Verification items for the finished model (mm, model axes). A direction names the side the tool comes from. Give positions to 0.01 mm unless a question says otherwise; leave off trailing zeros. Order: outer loops, then holes, each group sorted by start corner. A loop starts at its lowest first (then second) coordinate and runs counter-clockwise, first axis right, second up. Notation, with made-up numbers: M 43.5,79 L 72.5,79 A19 cw 72.5,108 Z; hole C 49,21.5 d9. An arc over 180 degrees is marked long. Answer as a JSON object with one key per item and string values.
```python
from build123d import *

# Parameters (mm, degrees)
BOSS_EXTRUDE1_DEPTH = 3


with BuildPart() as part:
    # Sketch1 → Boss-Extrude1 (new body)
    with BuildSketch(Plane(origin=(0, 0, 0), x_dir=(0, 0, -1), z_dir=(1, 0, 0))):
        Polygon((-23.405592815, -13.328738611), (32.192831055, -13.328738611), (32.192831055, -19.328738611), (34.462282484, -20.506092894), (31.699266712, -25.832042935), (36.137558413, -28.134556078), (38.900574185, -22.808606037), (44.171084966, -25.542860827), (41.408069194, -30.868810868), (45.846360891, -33.17132401), (48.609376663, -27.845373968), (53.879887443, -30.579628758), (51.116871671, -35.9055788), (55.555163369, -38.208091941), (58.318179141, -32.8821419), (60.336210887, -33.929063763), (60.336210887, -39.929063763), (60.336210887, -42.929063763), (50.45453087, -42.929063763), (50.45453087, -39.929063763), (10.850026953, -39.929063763), (10.850026953, -42.929063763), (5.387336757, -42.929063763), (5.387336757, -39.929063763), (5.387336757, -28.352747539), (-10.278235861, -19.965608879), (-23.405592815, -19.965608879), align=None)
    extrude(amount=BOSS_EXTRUDE1_DEPTH)


solid = part.part
```
Q1. Gauge pin test, flat ends, axial feed: pin 1 Ø1.5 at (x, z) = (1.5, -32) entering from -Y; pin 2 Ø1.5 at (x, y) = (1, -41) entering from +Z; pin 3 Ø1.5 at (x, y) = (1.5, -22.5) entering from +Z. Record the tip position at first contact, or that the pin passes through.
Resolved:
{"pin 1": "stops at y = -39.93", "pin 2": "stops at z = -5.39", "pin 3": "stops at z = 6.95"}
Q2. Tool access check on faces 5 (the face through (1.48, -23.13, -33.1)), 6 (the face through (1.479, -30.546, -47.209)), 7 (the face through (1, -16, -32.193)), 8 (the face through (1, -41, -50.455)). Record the directions out of +Z, -Z, +X, -X, +Y, -Y that give a thin tool (end or side, any length) a straight path to the whole face; none if there is none.
Resolved:
{"face 5": "+X, -X", "face 6": "+X, -X, +Y", "face 7": "-Z, +X, -X, +Y", "face 8": "+X, -X, -Y"}
Q3. Material ranges on L1, parallel to Y at x = 1.1, z = -27; L2, parallel to Z at x = 1.7, y = -25; L3, parallel to Z at x = 2.1, y = -32.5, recorded low to high.
Resolved:
{"L1": "y = -39.93 to -13.33", "L2": "z = -43.12 to -37.76, -32.13 to 0.87", "L3": "z = -52.88 to -46.19, -44.55 to -5.39"}
Q4. Section check A-A on y = -23.75. Record the cut outline in (x, z), then the cut area to 3 significant figures.
Resolved:
{"outline": "M 0,-40.72 L 3,-40.72 L 3,-38.41 L 0,-38.41 Z; M 0,-32.78 L 3,-32.78 L 3,3.21 L 0,3.21 Z", "area": "115 mm²"}
Q5. Section check B-B on x = 0.5. Record the cut outline in (y, z).
Resolved:
{"outline": "M -42.93,-60.34 L -33.93,-60.34 L -32.88,-58.32 L -38.21,-55.56 L -35.91,-51.12 L -30.58,-53.88 L -27.85,-48.61 L -33.17,-45.85 L -30.87,-41.41 L -25.54,-44.17 L -22.81,-38.9 L -28.13,-36.14 L -25.83,-31.7 L -20.51,-34.46 L -19.33,-32.19 L -13.33,-32.19 L -13.33,23.41 L -19.97,23.41 L -19.97,10.28 L -28.35,-5.39 L -42.93,-5.39 L -42.93,-10.85 L -39.93,-10.85 L -39.93,-50.45 L -42.93,-50.45 Z"}
Q6. Section check D-D on z = 18.5. Record the cut outline in (x, y), then the cut area to 3 significant figures.
Resolved:
{"outline": "M 0,-19.97 L 3,-19.97 L 3,-13.33 L 0,-13.33 Z", "area": "19.9 mm²"}
Q7. Release check for a two-part mould opening along Y. For faces 1 (the face through (1, -38, -60.336)), 2 (the face through (1, -42.929, -8)), 3 (the face through (1, -13.329, -4)), 4 (the face through (1.48, -26.97, -33.89)) record: +Y half, -Y half, draft (parallel to the pull), parting line (faces both ways), or undercut.
Resolved:
{"face 1": "draft", "face 2": "-Y half", "face 3": "+Y half", "face 4": "undercut"}
Q8. Section check C-C on z = -25. Record the cut outline in (x, y), then the cut area to 3 significant figures.
Resolved:
{"outline": "M 0,-39.93 L 3,-39.93 L 3,-13.33 L 0,-13.33 Z", "area": "79.8 mm²"}
